Autodesk Inventor part; units mm, degrees
ref_plane "YZ Plane" through (0, 0, 0) normal (1, 0, 0) x (0, 1, 0)
ref_plane "XZ Plane" through (0, 0, 0) normal (0, 1, 0) x (-1, 0, 0)
ref_plane "XY Plane" through (0, 0, 0) normal (0, 0, 1) x (1, 0, 0)
sketch "Skizze1" plane through (0, 0, 0) normal (0, 0, 1) x (1, 0, 0)
  line L0 (-7.5, 5.35) -> (-5.25, 5.35)
  line L1 (-5.25, 5.35) -> (-5.25, 6.55)
  line L2 (-5.25, 6.55) -> (-8.5, 6.55)
  line L3 (-8.5, 6.55) -> (-8.5, 0)
  line L4 (-8.5, 0) -> (0, 0)
  line L5 (0, 0) -> (0, 2.5)
  line L6 (-4.25, 3.75) -> (-7.5, 3.75)
  line L7 (-7.5, 3.75) -> (-7.5, 5.35)
  line L8 (0, 2.5) -> (-3, 2.5)
  line L9 (-3, 2.5) -> (-4.25, 3.75)
  dimension "d0" = 8.5
  dimension "d1" = 1.6
  dimension "d2" = 7.5
  dimension "d3" = 1.2
  dimension "d4" = 5.25
  dimension "d5" = 6.55
  dimension "d10" = 135
  dimension "d11" = 3
  dimension "d12" = 2.5
extrude "Extrusion1" add sketch "Skizze1" along normal blind 60
mirror "Spiegeln1" about plane through (0, 0, 0) normal (1, 0, 0) of "Extrusion1"
sketch "Skizze2" plane through (-3, 2.5, 60) normal (0, 1, 0) x (1, 0, 0)
  line L0 (3, 72) -> (3, -12)
  line L1 (0, 0) -> (6, 0)
  point P0 (3, 60)
  point P1 (3, 4)
  point P2 (3, 0)
  point P3 (3, 44)
  dimension "d13" = 4
  dimension "d14" = 40
hole "Bohrung1" at (0, 2.5, 56) at (0, 2.5, 16) direction (0, -1, 0) diameter 3.4 depth 2.5 countersink diameter 6.3 countersink angle 90
properties part number "igus_schine"
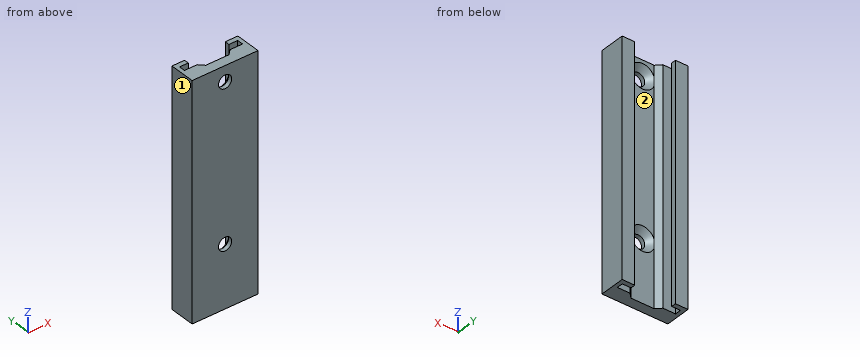
Read the model definition and answer for the solid it produces. Units are mm, in the model's axes. Face numbers are marked on the shaded views. A direction names the side the tool comes from. Give positions to 0.01 mm unless a question says otherwise; leave off trailing zeros. Loops run counter-clockwise (first coordinate to the right, second up) from the corner with the lowest first, then second, coordinate; pieces in that order, holes last. Notation, with made-up numbers: (-3.75, 79.5) -> (10.25, 79.5) arc R21 ccw to (10.25, 116.5) -> close; hole circle Ø10 at (43.25, 19.25). An arc over 180 degrees is marked (long way). Use a Markdown table: item, result.
Q1. Section C-C, the plane z = 16 is taken. Determine the outline of the cut face in (x, y), then the cut area to 3 significant figures.
Solved:
| item | result |
|---|---|
| outline | (-8.5, 0) -> (-1.7, 0) -> (-1.7, 1.05) -> (-3.15, 2.5) -> (-3, 2.5) -> (-4.25, 3.75) -> (-7.5, 3.75) -> (-7.5, 5.35) -> (-5.25, 5.35) -> (-5.25, 6.55) -> (-8.5, 6.55) -> close; (1.7, 0) -> (8.5, 0) -> (8.5, 6.55) -> (5.25, 6.55) -> (5.25, 5.35) -> (7.5, 5.35) -> (7.5, 3.75) -> (4.25, 3.75) -> (3, 2.5) -> (3.15, 2.5) -> (1.7, 1.05) -> close |
| area | 55.1 mm^2 |
Q2. Section A-A, the plane x = -6.5 is taken. Determine the outline of the cut face in (y, z).
Solved:
| item | result |
|---|---|
| outline | (0, 0) -> (3.75, 0) -> (3.75, 60) -> (0, 60) -> close; (5.35, 0) -> (6.55, 0) -> (6.55, 60) -> (5.35, 60) -> close |
Q3. Section B-B, the plane y = 1.75 is taken. Determine the outline of the cut face in (x, z), then the cut area to 3 significant figures.
Solved:
| item | result |
|---|---|
| outline | (-8.5, 0) -> (8.5, 0) -> (8.5, 60) -> (-8.5, 60) -> close; hole circle Ø4.8 at (0, 16); hole circle Ø4.8 at (0, 56) |
| area | 984 mm^2 |
Q4. Each of these flat-tipped pins is pushed along its axis until it touches: pin 1 (3 mm diameter, centred on x = 1, z = 8.5, fed in from +Y); pin 2 (6 mm diameter, centred on x = -1.5, z = 13, fed in from +Y). Where does it stop, or does it pass through?
Solved:
| item | result |
|---|---|
| pin 1 | stops at y = 2.5 |
| pin 2 | stops at y = 3.75 |
Q5. A tool of negligible diameter and unlimited length cuts with its end or side. For the marked faces 1 and 2, from which of +Z, -Z, +X, -X, +Y, -Y can it reach the whole face along a straight path? Write none if from no direction.
Solved:
| item | result |
|---|---|
| face 1 | +Z, -Z, -X, +Y, -Y |
| face 2 | +Z, -Z, +Y |
Q6. Section D-D, the plane x = 0 is taken. Determine the outline of the cut face in (y, z).
Solved:
| item | result |
|---|---|
| outline | (0, 0) -> (2.5, 0) -> (2.5, 12.85) -> (1.05, 14.3) -> (0, 14.3) -> close; (0, 17.7) -> (1.05, 17.7) -> (2.5, 19.15) -> (2.5, 52.85) -> (1.05, 54.3) -> (0, 54.3) -> close; (0, 57.7) -> (1.05, 57.7) -> (2.5, 59.15) -> (2.5, 60) -> (0, 60) -> close |
Q7. Find the intervals of material crossed by line 1 along Z through (x, y) = (0, 0.7); line 2 along X through (y, z) = (4.75, 42.5); line 3 along X through (y, z) = (0.3, 56), in increasing order.
Solved:
| item | result |
|---|---|
| line 1 | z = 0 to 14.3, 17.7 to 54.3, 57.7 to 60 |
| line 2 | x = -8.5 to -7.5, 7.5 to 8.5 |
| line 3 | x = -8.5 to -1.7, 1.7 to 8.5 |
